Can you work these out from the drawing? Everything is in mm from the part's minimum corner. A direction names the side the tool comes from. Coordinates: 2 decimals unless noted, no trailing zeros. Order: outer loops, then holes, each group sorted by start corner. A loop starts at its lowest first (then second) coordinate and runs counter-clockwise, first axis right, second up. Notation, with made-up numbers: (7.25, -16) - (37.25, -16) arc R14 ccw to (37.25, -10) - close; hole circle Ø9 at (67, 84). An arc over 180 degrees is marked (long way). One line per item, written item: value.
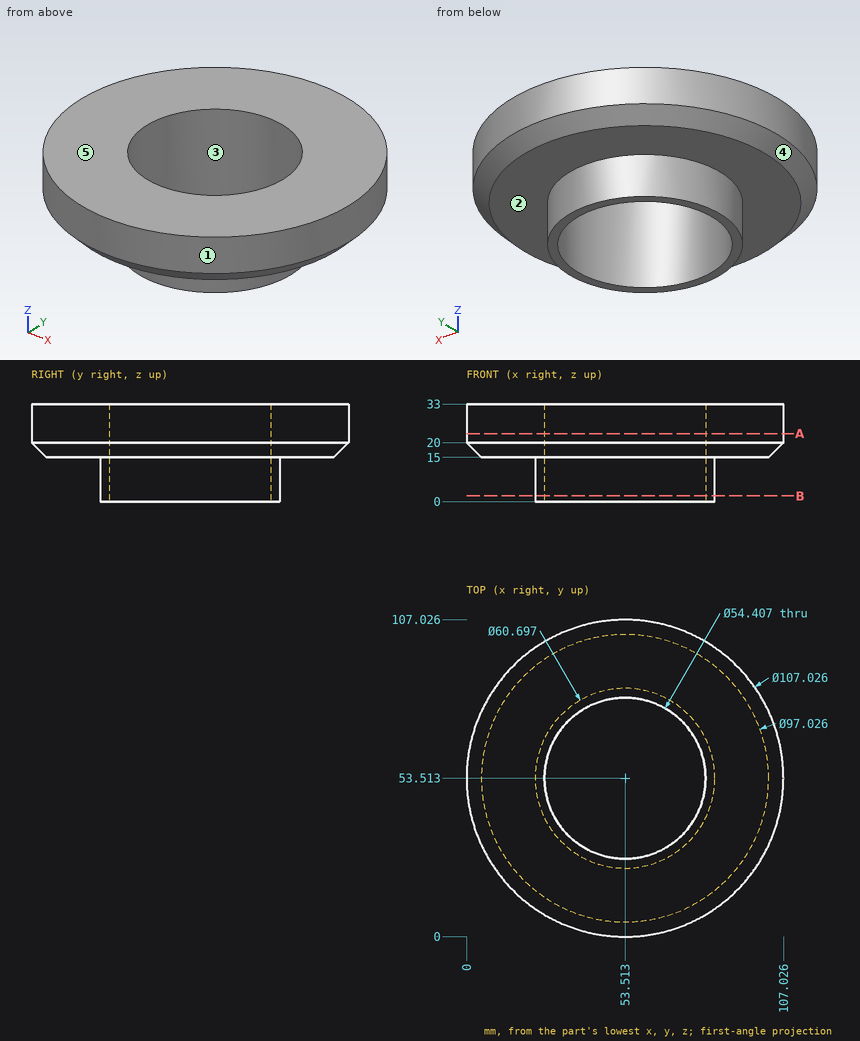
Item 1: Thinking about a two-plate mould opening in Y: for the marked faces 3, 4 and 5, which applies, pulls with the +Y half, pulls with the -Y half, needs draft (parallel to the pull), parting line crosses it, or undercut?
Conclusion:
face 3: undercut
face 4: parting line crosses it
face 5: needs draft
Item 2: I'm going to push flat-ended pins straight in: pin 1 Ø10 at (y, z) = (95.5, 11) entering from -X (1 decimal); pin 2 Ø5 at (x, z) = (24, 13.5) entering from -Y; pin 3 Ø6 at (y, z) = (85.5, 23.5) entering from -X. Where does each tip first touch, or does it pass through?
Conclusion:
pin 1: x = 24.6
pin 2: y = 13.27
pin 3: x = 8.53
Item 3: I want a section at A-A on z = 23. Please give me the cut outline in (x, y) (1 decimal).
Conclusion:
outline: circle Ø107 at (53.5, 53.5); hole circle Ø54.4 at (53.5, 53.5)
Item 4: If I drill on probe 1 along X at (y, z) = (48, 5); probe 2 along Y at (x, z) = (54, 5.5); probe 3 along X at (y, z) = (70.5, 26.5) (1 decimal), over which ranges is the centre line in solid material (lowest first)?
Conclusion:
probe 1: 23.67 to 26.87, 80.15 to 83.36
probe 2: 23.17 to 26.31, 80.71 to 83.86
probe 3: 2.8 to 32.3, 74.8 to 104.3
Item 5: For the marked faces 1 and 2, which set-ups out of +Z, -Z, +X, -X, +Y, -Y let a thin tool reach every point of the face, with its end or its side?
Conclusion:
face 1: +Z, -Z
face 2: -Z
Item 6: I want a section at B-B on z = 2. Please give me the cut outline in (x, y).
Conclusion:
outline: circle Ø60.7 at (53.51, 53.51); hole circle Ø54.41 at (53.51, 53.51)
